```python
from build123d import *

# Parameters (mm, degrees)
SKETCH_1_W          = 80
SKETCH_1_H          = 80
SKETCH_1_R          = 28
SKETCH_1_R_2        = 1.5
EXTRUDE_1_DEPTH     = 4
EXTRUDE_2_DEPTH     = 16
SKETCH_9_W          = 5
SKETCH_9_H          = 18
EXTRUDE_6_DEPTH     = 20
SKETCH_11_R         = 1.5
CUT_EXTRUDE_2_DEPTH = 80.14543575
CUT_EXTRUDE_START   = -1
SKETCH_12_R         = 35
SKETCH_12_R_2       = 28
CUT_EXTRUDE_3_DEPTH = 1
FILLET_6_R          = 10
SKETCH_13_R         = 1.5
CUT_EXTRUDE_4_DEPTH = 125.322162143
FILLET_8_R          = 2
SKETCH_15_W         = 5
SKETCH_15_H         = 18
CUT_EXTRUDE_6_DEPTH = 74.239333694
EXTRUDE_8_DEPTH     = 20
FILLET_9_R          = 2


with BuildPart() as part:
    # 草图1 → 凸台-拉伸1 (new body)
    with BuildSketch(Plane(origin=(0, 0, 0), x_dir=(1, 0, 0), z_dir=(0, 1, 0))):
        Rectangle(SKETCH_1_W, SKETCH_1_H)
        with Locations(Location((0, 0, 0), (0, 0, 270))):
            Circle(SKETCH_1_R, mode=Mode.SUBTRACT)
        with Locations(Location((0, 32, 0), (0, 0, 270))):
            Circle(SKETCH_1_R_2, mode=Mode.SUBTRACT)
        with Locations(Location((27.712812921, 16, 0), (0, 0, 270))):
            Circle(SKETCH_1_R_2, mode=Mode.SUBTRACT)
        with Locations(Location((27.712812921, -16, 0), (0, 0, 270))):
            Circle(SKETCH_1_R_2, mode=Mode.SUBTRACT)
        with Locations(Location((0, -32, 0), (0, 0, 270))):
            Circle(SKETCH_1_R_2, mode=Mode.SUBTRACT)
        with Locations(Location((-27.712812921, -16, 0), (0, 0, 270))):
            Circle(SKETCH_1_R_2, mode=Mode.SUBTRACT)
        with Locations(Location((-27.712812921, 16, 0), (0, 0, 270))):
            Circle(SKETCH_1_R_2, mode=Mode.SUBTRACT)
    extrude(amount=EXTRUDE_1_DEPTH)

    # 草图2 → 凸台-拉伸2 (add)
    with BuildSketch(Plane(origin=(0, 4, 0), x_dir=(1, 0, 0), z_dir=(0, 1, 0))):
        Polygon((40, 40), (-40, 40), (-40, 36.5), (-36.5, 36.5), (36.5, 36.5), (36.5, -36.5), (-36.5, -36.5), (-40, -36.5), (-40, -40), (40, -40), align=None)
    extrude(amount=EXTRUDE_2_DEPTH)

    # 草图9 → 凸台-拉伸6 (add)
    with BuildSketch(Plane(origin=(0, 20, 0), x_dir=(1, 0, 0), z_dir=(0, 1, 0))):
        with Locations((-7.5, -49)):
            Rectangle(SKETCH_9_W, SKETCH_9_H)
        with Locations((7.5, -49)):
            Rectangle(SKETCH_9_W, SKETCH_9_H)
        with Locations((7.5, 49)):
            Rectangle(SKETCH_9_W, SKETCH_9_H)
        with Locations((-7.5, 49)):
            Rectangle(SKETCH_9_W, SKETCH_9_H)
    extrude(amount=-EXTRUDE_6_DEPTH)

    # 草图11 → 切除-拉伸2 (cut, through all)
    with BuildSketch(Plane.ZY.offset(10)):
        with Locations((55, 15)):
            Circle(SKETCH_11_R)
        with Locations((55, 5)):
            Circle(SKETCH_11_R)
        with Locations((48, 5)):
            Circle(SKETCH_11_R)
        with Locations((48, 15)):
            Circle(SKETCH_11_R)
        with Locations(Location((-48, 15, 0), (0, 0, 180))):
            Circle(SKETCH_11_R)
        with Locations(Location((-48, 5, 0), (0, 0, 180))):
            Circle(SKETCH_11_R)
        with Locations(Location((-55, 5, 0), (0, 0, 180))):
            Circle(SKETCH_11_R)
        with Locations(Location((-55, 15, 0), (0, 0, 180))):
            Circle(SKETCH_11_R)
    extrude(amount=-CUT_EXTRUDE_2_DEPTH, mode=Mode.SUBTRACT)

    # 草图12 → 切除-拉伸3 (cut)
    with BuildSketch(Plane(origin=(0, 4, 0), x_dir=(1, 0, 0), z_dir=(0, 1, 0)).offset(CUT_EXTRUDE_START)):
        with Locations(Location((0, 0, 0), (0, 0, 270))):
            Circle(SKETCH_12_R)
        with Locations(Location((0, 0, 0), (0, 0, 270))):
            Circle(SKETCH_12_R_2, mode=Mode.SUBTRACT)
    extrude(amount=CUT_EXTRUDE_3_DEPTH, mode=Mode.SUBTRACT)

    # 圆角6
    fillet_6_edges = [part.edges().sort_by_distance(p)[0] for p in [
        (36.5, 12, -36.5),
        (36.5, 12, 36.5),
        (40, 10, -40),
        (40, 10, 40),
    ]]
    fillet(fillet_6_edges, radius=FILLET_6_R)

    # 草图13 → 切除-拉伸4 (cut, through all)
    with BuildSketch(Plane.XY.offset(58)):
        with Locations((-33.5, 7.5)):
            Circle(SKETCH_13_R)
        with Locations((-28, 7.5)):
            Circle(SKETCH_13_R)
        with Locations((-33.5, 15.5)):
            Circle(SKETCH_13_R)
        with Locations((-28, 15.5)):
            Circle(SKETCH_13_R)
    extrude(amount=-CUT_EXTRUDE_4_DEPTH, mode=Mode.SUBTRACT)

    # 圆角8
    fillet_8_edges = [part.edges().sort_by_distance(p)[0] for p in [
        (-40, 10, -40),
        (-40, 10, 40),
    ]]
    fillet(fillet_8_edges, radius=FILLET_8_R)

    # 草图15 → 切除-拉伸6 (cut, through all)
    with BuildSketch(Plane(origin=(0, 20, 0), x_dir=(1, 0, 0), z_dir=(0, 1, 0))):
        with Locations((-7.5, -49)):
            Rectangle(SKETCH_15_W, SKETCH_15_H)
        with Locations((-7.5, 49)):
            Rectangle(SKETCH_15_W, SKETCH_15_H)
    extrude(amount=-CUT_EXTRUDE_6_DEPTH, mode=Mode.SUBTRACT)

    # 草图16 → 凸台-拉伸8 (add)
    with BuildSketch(Plane(origin=(0, 20, 0), x_dir=(1, 0, 0), z_dir=(0, 1, 0))):
        Polygon((10, -42), (25, -40), (10, -40), align=None)
        Polygon((5, -42), (5, -40), (-10, -40), align=None)
        Polygon((10, 42), (10, 40), (25, 40), align=None)
        Polygon((5, 42), (-10, 40), (5, 40), align=None)
    extrude(amount=-EXTRUDE_8_DEPTH)

    # 圆角9
    fillet_9_edges = [part.edges().sort_by_distance(p)[0] for p in [
        (10, 10, 42),
        (5, 10, 42),
        (10, 10, -42),
        (5, 10, -42),
    ]]
    fillet(fillet_9_edges, radius=FILLET_9_R)


solid = part.part
```
Input: part model. Units: mm. Frame: model coordinates. A direction names the side the tool comes from. Give positions to 0.01 mm unless a question says otherwise; leave off trailing zeros. Loops run counter-clockwise (first coordinate to the right, second up) from the corner with the lowest first, then second, coordinate; pieces in that order, holes last.
1) Contact query for flat-ended pins moving along their axis: pin 1 (12 mm diameter, centred on x = -18.5, y = 8, fed in from -Z); pin 2 (12 mm diameter, centred on x = -8, y = 8, fed in from -Z); pin 3 (1.8 mm diameter, centred on x = -28, y = 15.5, fed in from +Z); pin 4 (11.5 mm diameter, centred on y = 15, z = -48, fed in from +X). Output: stop coordinate, or through.
A:
pin 1: stops at z = -40
pin 2: stops at z = -41.07
pin 3: passes through
pin 4: stops at x = 10.68
2) Reachability of faces 4 (the flat face through (-24, 10, 40)), 5 (the cylindrical face through (-21.3, 3.49, -27.77)), 6 (the flat face through (-24, 10, -40)), 7 (the flat face through (10, 10, 51)) from +Z, -Z, +X, -X, +Y, -Y: full face, straight path, thin tool, end or side. Return the list, or none.
A:
face 4: +Z, -X, +Y, -Y
face 5: +Y
face 6: -Z, -X, +Y, -Y
face 7: +Z, +X, +Y, -Y
3) Mould query, pull axis Y, two halves, no side actions, for faces 1 (the flat face through (28, 10, -40)), 2 (the cylindrical face through (-29.5, 15.57, -38.23)), 3 (the flat face through (-36, 4, 3)). Classes: released by +Y, released by -Y, zero draft, split by the parting line, or undercut.
A:
face 1: zero draft
face 2: undercut
face 3: released by +Y
4) Line query: L1, parallel to Y at x = -33.5, z = 39.15; L2, parallel to Y at x = 8.4, z = -48; L3, parallel to Z at x = -21, y = 12.5. Output: solid intervals per line, ascending.
A:
L1: y = 0 to 6, 9 to 14, 17 to 20
L2: y = 0 to 3.5, 6.5 to 13.5, 16.5 to 20
L3: z = -40 to -36.5, 36.5 to 40
5) Section query A-A on z = -55. Return the cut outline in (x, y), and give its area (3 significant figures).
A:
outline: (5, 0) - (10, 0) - (10, 3.5) - (5, 3.5) - close; (5, 6.5) - (10, 6.5) - (10, 13.5) - (5, 13.5) - close; (5, 16.5) - (10, 16.5) - (10, 20) - (5, 20) - close
area: 70.0 mm2
6) Section query D-D on z = 13. Return the cut outline in (x, y), and give its area (3 significant figures).
A:
outline: (-40, 0) - (-24.8, 0) - (-24.8, 3) - (-32.5, 3) - (-32.5, 4) - (-40, 4) - close; (24.8, 0) - (40, 0) - (40, 20) - (36.5, 20) - (36.5, 4) - (32.5, 4) - (32.5, 3) - (24.8, 3) - close
area: 162 mm2
7) Section query C-C on x = -33.5. Return the cut outline in (y, z), and give its area (3 significant figures).
A:
outline: (0, -40) - (6, -40) - (6, -36.5) - (4, -36.5) - (4, -10.14) - (3, -10.14) - (3, 10.14) - (4, 10.14) - (4, 36.5) - (6, 36.5) - (6, 40) - (0, 40) - close; (9, -40) - (14, -40) - (14, -36.5) - (9, -36.5) - close; (9, 36.5) - (14, 36.5) - (14, 40) - (9, 40) - close; (17, -40) - (20, -40) - (20, -36.5) - (17, -36.5) - close; (17, 36.5) - (20, 36.5) - (20, 40) - (17, 40) - close
area: 370 mm2
8) Section query B-B on z = 32. Return the cut outline in (x, y), and give its area (3 significant figures).
A:
outline: (-40, 0) - (-1.5, 0) - (-1.5, 3) - (-14.18, 3) - (-14.18, 4) - (-40, 4) - close; (1.5, 0) - (39.8, 0) - (39.8, 20) - (34.85, 20) - (34.85, 4) - (14.18, 4) - (14.18, 3) - (1.5, 3) - close
area: 361 mm2
